Verification items for the finished model (mm, model axes). Round coordinates to 2 decimals unless told otherwise and drop trailing zeros. Write each loop counter-clockwise with the first axis right and the second up, starting at its lowest first coordinate (ties: lowest second). Pieces come first, ordered by that corner, then holes. Notation, with made-up numbers: (-34.75, -12.75) -> (-7.75, -12.75) arc R27 cw to (-7.75, 17.25) -> close; hole circle Ø8 at (20.25, 68.5). An arc over 180 degrees is marked (long way). Answer as a JSON object with one key per item and string values. Group by question number.
(1) Scan lines: L1, parallel to X at y = 2.35, z = 94 (3 decimals); L2, parallel to Z at x = 86, y = 2.85; L3, parallel to Z at x = -18.5, y = 0.8 (3 decimals). Record each from-to range of solid material in increasing order. Write a range as from..to.
(2) Gauge pin test, flat ends, axial feed: pin 1 Ø2.5 at (x, z) = (-78.97, -93.59) entering from +Y; pin 2 Ø1 at (x, y) = (115.5, 1) entering from +Z; pin 3 Ø1 at (x, y) = (-1.5, 2) entering from -Z (3 decimals). Record the tip position at first contact, or that the pin passes through.
(3) Sectioned sample at C-C on x = -129.5. Record the cut outline in (y, z) (1 decimal).
(4) Sectioned sample at B-B on x = -7. Record the cut outline in (y, z) (3 decimals).
(5) Sectioned sample at A-A on y = 0.9. Record the cut outline in (x, z) (3 decimals), and give its area (4 significant figures).
Autodesk Inventor part; units mm, degrees
ref_plane "YZ Plane" through (0, 0, 0) normal (1, 0, 0) x (0, 1, 0)
ref_plane "XZ Plane" through (0, 0, 0) normal (0, 1, 0) x (-1, 0, 0)
ref_plane "XY Plane" through (0, 0, 0) normal (0, 0, 1) x (1, 0, 0)
sketch "Sketch1" plane through (0, 0, 0) normal (0, 1, 0) x (-1, 0, 0)
  line L0 (149.225, -123.825) -> (-149.225, -123.825)
  line L1 (-149.225, -123.825) -> (-149.225, 123.825)
  line L2 (-149.225, 123.825) -> (149.225, 123.825)
  line L3 (149.225, 123.825) -> (149.225, -123.825)
  line L4 (149.225, -123.825) -> (-149.225, 123.825) construction
  line L5 (-149.225, -123.825) -> (149.225, 123.825) construction
  point P0 (0, 0)
  dimension "d0" = 298.45
  dimension "d1" = 247.65
extrude "Extrusion1" add sketch "Sketch1" along normal blind 3.175
sketch "Sketch2" plane through (0, 3.175, 0) normal (0, 1, 0) x (1, 0, 0)
  line L0 (149.225, 123.825) -> (-149.225, 123.825)
  line L1 (-149.225, 123.825) -> (-149.225, -123.825)
  line L2 (-149.225, -123.825) -> (149.225, -123.825)
  line L3 (149.225, -123.825) -> (149.225, 123.825)
  line L4 (-149.225, 104.775) -> (-85.725, 123.825)
  line L5 (85.725, 123.825) -> (149.225, 104.775)
  line L6 (149.225, -104.775) -> (85.725, -123.825)
  line L7 (-85.725, -123.825) -> (-149.225, -104.775)
  point P0 (0, 0)
  dimension "d4" = 19.05
  dimension "d5" = 19.05
  dimension "d6" = 19.05
  dimension "d7" = 19.05
  dimension "d8" = 63.5
  dimension "d9" = 63.5
  dimension "d10" = 63.5
extrude "Extrusion2" cut sketch "Sketch2" against normal blind 3.175 contours L3 L5 L0 | L4 L1 L0 | L3 L2 L6 | L7 L2 L1
sketch "Sketch3" plane through (0, 3.175, 0) normal (0, 1, 0) x (1, 0, 0)
  line L0 (85.725, 123.825) -> (-85.725, 123.825)
  line L1 (-38.1, 123.825) -> (38.1, 123.825)
  line L2 (38.1, 123.825) -> (38.1, 85.725)
  line L3 (38.1, 85.725) -> (-38.1, 85.725)
  line L4 (-38.1, 85.725) -> (-38.1, 123.825)
  point P0 (0, 0)
  point P1 (0, 85.725)
  dimension "d13" = 38.1
  dimension "d14" = 76.2
extrude "Extrusion3" cut sketch "Sketch3" against normal blind 3.175
fillet "Fillet1" radius 3.175 12 edges at (38.1, 1.5875, -85.725) (-38.1, 1.5875, -85.725) (38.1, 1.5875, -123.825) (-38.1, 1.5875, -123.825) (85.725, 1.5875, -123.825) (-85.725, 1.5875, -123.825) (-149.225, 1.5875, -104.775) (149.225, 1.5875, -104.775) (-149.225, 1.5875, 104.775) (-85.725, 1.5875, 123.825) (85.725, 1.5875, 123.825) (149.225, 1.5875, 104.775)
sketch "Sketch4" plane through (0, 3.175, 0) normal (0, 1, 0) x (1, 0, 0)
  point P0 (0, 0)
  point P1 (-78.9686, 93.5863)
  point P2 (-78.9686, -93.5863)
  point P3 (78.9686, -93.5863)
  point P4 (78.9686, 93.5863)
  dimension "d18" = 93.5863
  dimension "d19" = 93.5863
  dimension "d20" = 78.9686
  dimension "d21" = 78.9686
hole "Hole1" at (-78.9686, 3.175, -93.5863) at (-78.9686, 3.175, 93.5863) at (78.9686, 3.175, 93.5863) at (78.9686, 3.175, -93.5863) direction (0, -1, 0) diameter 3.302 end through all
properties part number "SwarmieCoverPlate"
Computed values:
{
 "1": {"L1": "-149.225..-80.567, -77.37..77.37, 80.567..149.225", "L2": "-123.74..123.74", "L3": "-85.725..123.825"},
 "2": {"pin 1": "through", "pin 2": "z = 115.04", "pin 3": "z = -85.725"},
 "3": {"outline": "(0, -110.7) -> (3.2, -110.7) -> (3.2, 110.7) -> (0, 110.7) -> close"},
 "4": {"outline": "(0, -85.725) -> (3.175, -85.725) -> (3.175, 123.825) -> (0, 123.825) -> close"},
 "5": {"outline": "(-149.225, -102.413) arc R3.175 ccw to (-146.962, -105.454) -> (-86.171, -123.691) arc R3.175 ccw to (-85.259, -123.825) -> (-41.275, -123.825) arc R3.175 ccw to (-38.1, -120.65) -> (-38.1, -88.9) arc R3.175 cw to (-34.925, -85.725) -> (34.925, -85.725) arc R3.175 cw to (38.1, -88.9) -> (38.1, -120.65) arc R3.175 ccw to (41.275, -123.825) -> (85.259, -123.825) arc R3.175 ccw to (86.171, -123.691) -> (146.962, -105.454) arc R3.175 ccw to (149.225, -102.413) -> (149.225, 102.413) arc R3.175 ccw to (146.962, 105.454) -> (86.171, 123.691) arc R3.175 ccw to (85.259, 123.825) -> (-85.259, 123.825) arc R3.175 ccw to (-86.171, 123.691) -> (-146.962, 105.454) arc R3.175 ccw to (-149.225, 102.413) -> close; hole circle Ø3.302 at (-78.969, -93.586); hole circle Ø3.302 at (-78.969, 93.586); hole circle Ø3.302 at (78.969, -93.586); hole circle Ø3.302 at (78.969, 93.586)", "area": "68,550 mm2"}
}
